Could you check a few things on this model? Use its own coordinates, in mm. A direction names the side the tool comes from. Give positions to 0.01 mm unless a question says otherwise; leave off trailing zeros. Loops run counter-clockwise (first coordinate to the right, second up) from the corner with the lowest first, then second, coordinate; pieces in that order, holes last. Notation, with made-up numbers: M 19,0 L 32,0 A17 cw 32,22 Z; hole C 38.25,-2 d1. An arc over 180 degrees is marked long. Use a Markdown table: item, result. Add a question column.
1) Will these pins go through, and if not, where does the flat tip stop? pin 1 Ø1 at (y, z) = (4, 3.5) entering from -X; pin 2 Ø2.5 at (x, y) = (-0.5, -8.5) entering from +Z; pin 3 Ø12 at (x, y) = (-2, 9) entering from -Z; pin 4 Ø8 at (x, y) = (-0.5, 9) entering from +Z.
2) If I drill on line 1 along X through (y, z) = (-5.5, 6); line 2 along Z through (x, y) = (-13.5, -5.5); line 3 along X through (y, z) = (-15.5, 2), over which ranges is the centre line in solid material (lowest first)? Write a range as [from, to].
3) Suppose I cut it at D-D on z = 3.5. Count the separate pieces of the cut face and the enclosed holes in it, and give its area (3 significant figures).
4) Suppose I cut it at B-B on y = 7.5. List the corners of the cut face in (x, z) for me, and give its area (3 significant figures).
5) Which directions (+Z, -Z, +X, -X, +Y, -Y) give clear straight access to the entire face, cutting with the end or side of a thin tool? Please do faces 1 (the flat face through (-14, -7, 6.604)), 2 (the flat face through (0, -4.699, 3)), 3 (the flat face through (-15, -6.998, 4)), 4 (the flat face through (-3, -18, 0.508)).
6) Suppose I cut it at A-A on z = 6. List the corners of the cut face in (x, y) for me, and give its area (3 significant figures).
7) We'd pull the mould along X, two halves only. Please class faces 5 (the cylindrical face through (20.543, -7.501, 3.789)), 6 (the cylindrical face through (-20.543, -7.501, 3.789)), 7 (the flat face through (-2.159, 4, 3)), 8 (the flat face through (14, -4.966, 6)): +X half, -X half, draft (parallel to the pull), parting line (faces both ways), or undercut.
```python
from build123d import *

# Parameters (mm, degrees)
F1_ANGLE  = 90
F3_DEPTH  = 25.4
F4_DEPTH  = 0.762
F6_DEPTH  = 3.048
F7_W      = 9.631022
F7_H      = 1.778
F8_DEPTH  = 3.048
F9_W      = 2.159
F9_H      = 1.2065
F10_DEPTH = 2.9972
F13_R     = 2.2098
F13_R_2   = 1.0668
F14_DEPTH = 3.683
F15_SIZE  = 0.508


with BuildPart() as f1:
    # F0 (on Front) → F1 (revolve)
    with BuildSketch(Plane.XZ):
        Polygon((-17.907, 0), (0, 0), (0, 1.524), (-19.0246, 1.524), (-19.0246, 7.112), (-20.0406, 7.112), (-20.0406, 1.524), (-20.8534, 1.524), (-20.8534, 5.334), (-21.8694, 5.334), (-21.8694, 0), (-19.8628, 0), (-19.8628, 0.508), (-17.907, 0.508), align=None)
    revolve(axis=Axis((0, 0, 5.251978), (0, 0, 1)), revolution_arc=F1_ANGLE)

    # F2 (on face) → F3 (cut)
    with BuildSketch(Plane.XY.offset(1.524)):
        with BuildLine():
            Line((0, -3.4925), (0, -2.4257))
            Line((0, -2.4257), (-8.7376, -2.4257))
            Line((-8.7376, -2.4257), (-8.7376, 0))
            Line((-8.7376, 0), (-21.8694, 0))
            ThreePointArc((-21.8694, 0), (-21.485747, -4.078397), (-20.34825, -8.0137))
            Line((-20.34825, -8.0137), (-8.7376, -8.0137))
            Line((-8.7376, -8.0137), (-8.7376, -3.4925))
            Line((-8.7376, -3.4925), (0, -3.4925))
        make_face()
    extrude(amount=F3_DEPTH, mode=Mode.SUBTRACT)

    # F2 (on face) → F4 (join)
    with BuildSketch(Plane.XY.offset(1.524)):
        with BuildLine():
            Line((0, -3.4925), (0, -2.4257))
            Line((0, -2.4257), (-8.7376, -2.4257))
            Line((-8.7376, -2.4257), (-8.7376, 0))
            Line((-8.7376, 0), (-21.8694, 0))
            ThreePointArc((-21.8694, 0), (-21.485747, -4.078397), (-20.34825, -8.0137))
            Line((-20.34825, -8.0137), (-8.7376, -8.0137))
            Line((-8.7376, -8.0137), (-8.7376, -3.4925))
            Line((-8.7376, -3.4925), (0, -3.4925))
        make_face()
    extrude(amount=F4_DEPTH)

    # F5 (on face) → F6 (join, through all)
    with BuildSketch(Plane.XY.offset(2.286)):
        with BuildLine():
            Line((-20.34825, -8.0137), (-8.7376, -8.0137))
            Line((-8.7376, -8.0137), (-8.7376, -6.9977))
            Line((-8.7376, -6.9977), (-20.719625, -6.9977))
            ThreePointArc((-20.719625, -6.9977), (-20.54022, -7.507997), (-20.34825, -8.0137))
        make_face()
    extrude(amount=F6_DEPTH)

    # F7 (on face) → F8 (join)
    with BuildSketch(Plane.XZ.offset(8.0137)):
        with Locations((-13.553111, 5.715)):
            Rectangle(F7_W, F7_H)
    extrude(amount=-F8_DEPTH)

    # F9 (on face) → F10 (join)
    with BuildSketch(Plane.XY.offset(1.524)):
        with Locations((-1.0795, -4.09575)):
            Rectangle(F9_W, F9_H)
    extrude(amount=F10_DEPTH)

    # F11: F1 across face


with BuildPart() as f1_1:
    add(f1.part)
    add(f1.part.mirror(Plane(origin=(0, -12.015662, 1.628309), x_dir=(0, 1, 0), z_dir=(1, 0, 0))))

    # F12: F1 across face


with BuildPart() as f1_2:
    add(f1_1.part)
    add(f1_1.part.mirror(Plane(origin=(0, 0, 1.044039), x_dir=(-1, 0, 0), z_dir=(0, 1, 0))))

    # F13 (on face) → F14 (join)
    with BuildSketch(Plane.XY.offset(1.524)):
        with Locations((0, -7.8867)):
            Circle(F13_R)
        with Locations((0, -7.8867)):
            Circle(F13_R_2, mode=Mode.SUBTRACT)
    extrude(amount=F14_DEPTH)

    # F15
    f15_edges = [f1_2.edges().sort_by_distance(p)[0] for p in [
        (-2.2098, -7.8867, 5.207),
    ]]
    chamfer(f15_edges, length=F15_SIZE)


solid = f1_2.part
```
Answer block:
| question | item | result |
|---|---|---|
| 1 | pin 1 | stops at x = -2.16 |
| 1 | pin 2 | stops at z = 5.21 |
| 1 | pin 3 | stops at z = 0 |
| 1 | pin 4 | stops at z = 1.52 |
| 2 | line 1 | x = [-18.37, -8.74], [8.74, 18.37] |
| 2 | line 2 | z = [0, 2.29], [4.83, 6.6] |
| 2 | line 3 | x = [-15.43, -13.95], [-12.7, -11.03], [11.03, 12.7], [13.95, 15.43] |
| 3 | separate pieces | 5 |
| 3 | enclosed holes | 3 |
| 3 | area | 264 mm^2 |
| 4 | outline | M -20.54,0 L -18.39,0 L -18.39,0.51 L -16.26,0.51 L -16.26,0 L 16.26,0 L 16.26,0.51 L 18.39,0.51 L 18.39,0 L 20.54,0 L 20.54,5.33 L 18.37,5.33 L 18.37,6.6 L 8.74,6.6 L 8.74,1.52 L -8.74,1.52 L -8.74,6.6 L -18.37,6.6 L -18.37,5.33 L -20.54,5.33 Z |
| 4 | area | 175 mm^2 |
| 5 | face 1 | +Z, +X, -X |
| 5 | face 2 | +Z |
| 5 | face 3 | -X |
| 5 | face 4 | -Z |
| 6 | outline | M -18.37,-8.01 A20.04 ccw 18.37,-8.01 L 18.37,-4.97 L 8.74,-4.97 L 8.74,-8.01 L 17.25,-8.01 A19.02 cw -17.25,-8.01 L -8.74,-8.01 L -8.74,-4.97 L -18.37,-4.97 Z; M -18.37,4.97 L -8.74,4.97 L -8.74,8.01 L -17.25,8.01 A19.02 cw 17.25,8.01 L 8.74,8.01 L 8.74,4.97 L 18.37,4.97 L 18.37,8.01 A20.04 ccw -18.37,8.01 Z |
| 6 | area | 209 mm^2 |
| 7 | face 5 | +X half |
| 7 | face 6 | -X half |
| 7 | face 7 | undercut |
| 7 | face 8 | draft |
